Part model, mm, in its own coordinate system. Face numbers are marked on the shaded views. A direction names the side the tool comes from. Give positions to 0.01 mm unless a question says otherwise; leave off trailing zeros. Order: outer loops, then holes, each group sorted by start corner. A loop starts at its lowest first (then second) coordinate and runs counter-clockwise, first axis right, second up. Notation, with made-up numbers: M 9,-38 L 46,-38 A18 ccw 46,-9 Z; hole C 12.5,52.5 d4. An arc over 180 degrees is marked long. Return JSON: item names as keys, results as strings.
from build123d import *

# Parameters (mm, degrees)
CROQUIS1_R                   = 11
SALIENTE_EXTRUIR1_DEPTH      = 5
SALIENTE_EXTRUIR2_START      = 6
CROQUIS2_R                   = 11
SALIENTE_EXTRUIR2_DEPTH      = 6
CROQUIS3_R                   = 2.25
CORTAR_EXTRUIR1_DEPTH        = 20.052558883
SALIENTE_EXTRUIR3_DEPTH      = 5
SALIENTE_EXTRUIR3_DEPTH_BACK = 5
SALIENTE_EXTRUIR4_DEPTH      = 10
CROQUIS6_R                   = 2.25
CORTAR_EXTRUIR2_DEPTH        = 130.193653111
CROQUIS7_R                   = 10.9
CORTAR_EXTRUIR3_DEPTH        = 7
CROQUIS8_R                   = 4.25
CORTAR_EXTRUIR4_DEPTH        = 129.740048173
CROQUIS9_R                   = 2.5
CORTAR_EXTRUIR5_DEPTH        = 130.193653111


with BuildPart() as part:
    # Croquis1 → Saliente-Extruir1 (new, symmetric)
    with BuildSketch(Plane.XY):
        Circle(CROQUIS1_R)
        with BuildLine():
            Line((1.833030278, 2.5), (-1.833030278, 2.5))
            ThreePointArc((-1.833030278, 2.5), (0, -3.1), (1.833030278, 2.5))
        make_face(mode=Mode.SUBTRACT)
    extrude(amount=SALIENTE_EXTRUIR1_DEPTH, both=True)

    # Croquis2 → Saliente-Extruir2 (add)
    with BuildSketch(Plane.XY.offset(5).offset(SALIENTE_EXTRUIR2_START)):
        Circle(CROQUIS2_R)
    extrude(amount=-SALIENTE_EXTRUIR2_DEPTH)

    # Croquis3 → Cortar-Extruir1 (cut, through all)
    with BuildSketch(Plane(origin=(0, 0, 0), x_dir=(1, 0, 0), z_dir=(0, 1, 0))):
        with Locations(Location((0, 0, 0), (0, 0, 90))):
            Circle(CROQUIS3_R)
    extrude(amount=CORTAR_EXTRUIR1_DEPTH, mode=Mode.SUBTRACT)

    # Croquis4 → Saliente-Extruir3 (add, two sides: drawn at the far end of the back side and taken through both)
    with BuildSketch(Plane.XY.offset(11).offset(-SALIENTE_EXTRUIR3_DEPTH_BACK)):
        with BuildLine():
            Line((-25, 0), (-25, -85))
            Line((-25, -85), (25, -85))
            Line((25, -85), (25, 0))
            ThreePointArc((25, 0), (0, 25), (-25, 0))
        make_face()
    extrude(amount=SALIENTE_EXTRUIR3_DEPTH + SALIENTE_EXTRUIR3_DEPTH_BACK)

    # Croquis5 → Saliente-Extruir4 (add)
    with BuildSketch(Plane.XY.offset(16)):
        with BuildLine():
            Line((-25, -100), (-25, -85))
            Line((-25, -85), (25, -85))
            Line((25, -85), (25, -100))
            ThreePointArc((25, -100), (0, -125), (-25, -100))
        make_face()
    extrude(amount=-SALIENTE_EXTRUIR4_DEPTH)

    # Croquis6 → Cortar-Extruir2 (cut, through all)
    with BuildSketch(Plane.XY.offset(16)):
        with Locations((0, -35)):
            Circle(CROQUIS6_R)
        with Locations((0, -65)):
            Circle(CROQUIS6_R)
    extrude(amount=-CORTAR_EXTRUIR2_DEPTH, mode=Mode.SUBTRACT)

    # Croquis7 → Cortar-Extruir3 (cut)
    with BuildSketch(Plane(origin=(0, 0, 6), x_dir=(-1, 0, 0), z_dir=(0, 0, -1))):
        with Locations((0, -100)):
            Circle(CROQUIS7_R)
    extrude(amount=-CORTAR_EXTRUIR3_DEPTH, mode=Mode.SUBTRACT)

    # Croquis8 → Cortar-Extruir4 (cut, through all)
    with BuildSketch(Plane(origin=(0, 0, 13), x_dir=(-1, 0, 0), z_dir=(0, 0, -1))):
        with Locations((0, -100)):
            Circle(CROQUIS8_R)
    extrude(amount=-CORTAR_EXTRUIR4_DEPTH, mode=Mode.SUBTRACT)

    # Croquis9 → Cortar-Extruir5 (cut, through all)
    with BuildSketch(Plane.XY.offset(16)):
        with Locations((17.95, -100)):
            Circle(CROQUIS9_R)
    extrude(amount=-CORTAR_EXTRUIR5_DEPTH, mode=Mode.SUBTRACT)


solid = part.part
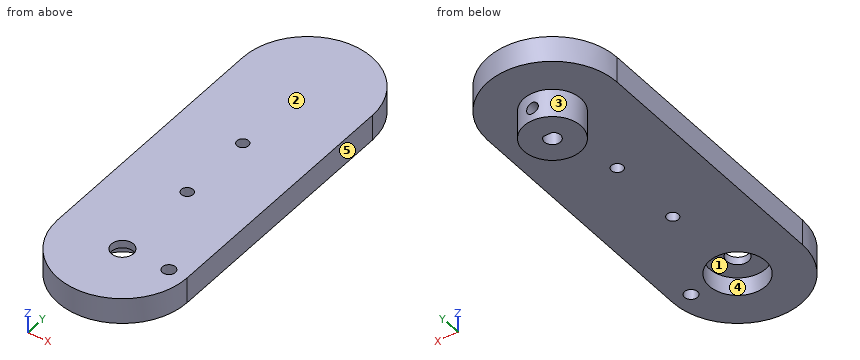
Q1. Band-saw the part on A-A (z = 9). Give the cut face in (x, y).
Established:
{"outline": "M -25,-100 A25 ccw 25,-100 L 25,0 A25 ccw -25,0 Z; hole C 0,-100 d21.8; hole C 0,-65 d4.5; hole C 0,-35 d4.5; hole C 17.95,-100 d5"}
Q2. Band-saw the part on C-C (x = 0). Give the number of separate pieces and of enclosed holes in the cut face, then the cut area to 3 significant figures.
Established:
{"separate pieces": "5", "enclosed holes": "0", "area": "1,380 mm²"}
Q3. Two-plate mould, pull along X, no slides. Class the marked faces 1, 2 and 3: +X half, -X half, draft (parallel to the pull), parting line (faces both ways), or undercut.
Established:
{"face 1": "undercut", "face 2": "draft", "face 3": "parting line"}
Q4. 3-axis set-ups, long thin cutter, end or side, ignore diameter. For the marked faces 4 and 5: which of +Z, -Z, +X, -X, +Y, -Y reach the whole face in a straight line?
Established:
{"face 4": "-Z", "face 5": "+Z, -Z, +X, +Y, -Y"}
Q5. Probe line 1 along Y through (x, z) = (0, 8); line 2 along Z through (x, y) = (15, -101); line 3 along Y through (x, z) = (1, 14.75). List the from-to ranges inside material, lowest first.
Established:
{"line 1": "y = -125 to -110.9, -89.1 to -67.25, -62.75 to -37.25, -32.75 to 25", "line 2": "z = 6 to 16", "line 3": "y = -124.98 to -104.13, -95.87 to -67.02, -62.98 to -37.02, -32.98 to 24.98"}
Q6. Band-saw the part on B-B (y = -65). Give the cut face in (x, z).
Established:
{"outline": "M -25,6 L -2.25,6 L -2.25,16 L -25,16 Z; M 2.25,6 L 25,6 L 25,16 L 2.25,16 Z"}
Q7. Band-saw the part on D-D (x = 17.95). Give the cut face in (y, z).
Established:
{"outline": "M -117.4,6 L -102.5,6 L -102.5,16 L -117.4,16 Z; M -97.5,6 L 17.4,6 L 17.4,16 L -97.5,16 Z"}
Q8. Pin check, flat tips, straight feed: pin 1 (1.8 mm diameter, centred on x = 1, z = 2.5, fed in from -Y); pin 2 (4 mm diameter, centred on x = 0, z = 0, fed in from +Y); pin 3 (4 mm diameter, centred on x = 9.5, y = -79, fed in from -Z). Stop position of each tip, or through.
Established:
{"pin 1": "stops at y = -11", "pin 2": "stops at y = -2.37", "pin 3": "stops at z = 6"}
